```python
from build123d import *

# Parameters (mm, degrees)
SKETCH1_W           = 17
SKETCH1_H           = 10
BOSS_EXTRUDE1_DEPTH = 1
SKETCH2_W           = 3
SKETCH2_H           = 4
BOSS_EXTRUDE2_DEPTH = 1
SKETCH3_W           = 22.308498818
SKETCH3_H           = 11.48116176
SKETCH3_W_2         = 12.6
SKETCH3_H_2         = 7.6
CUT_EXTRUDE1_DEPTH  = 1
SKETCH4_R           = 0.5
SKETCH4_R_2         = 1.1
CUT_EXTRUDE2_DEPTH  = 1
SKETCH5_W           = 3.647171716
SKETCH5_H           = 4.834622973
SKETCH5_W_2         = 2.9
SKETCH5_H_2         = 3.6
CUT_EXTRUDE3_DEPTH  = 1


with BuildPart() as part:
    # Sketch1 → Boss-Extrude1 (new body)
    with BuildSketch(Plane(origin=(0, 0, 0), x_dir=(1, 0, 0), z_dir=(0, 1, 0))):
        with Locations((-16, 13.384146341)):
            Rectangle(SKETCH1_W, SKETCH1_H)
    extrude(amount=BOSS_EXTRUDE1_DEPTH)

    # Sketch2 → Boss-Extrude2 (add)
    with BuildSketch(Plane(origin=(0, 1, 0), x_dir=(1, 0, 0), z_dir=(0, 1, 0))):
        with Locations((-21, 13.384146341)):
            Rectangle(SKETCH2_W, SKETCH2_H)
    extrude(amount=BOSS_EXTRUDE2_DEPTH)

    # Sketch3 → Cut-Extrude1 (cut)
    with BuildSketch(Plane(origin=(0, 1, 0), x_dir=(1, 0, 0), z_dir=(0, 1, 0))):
        with Locations((-18.026856575, 13.593370246)):
            Rectangle(SKETCH3_W, SKETCH3_H)
        with Locations((-18.2, 13.384146341)):
            Rectangle(SKETCH3_W_2, SKETCH3_H_2, mode=Mode.SUBTRACT)
    extrude(amount=-CUT_EXTRUDE1_DEPTH, mode=Mode.SUBTRACT)

    # Sketch4 → Cut-Extrude2 (cut)
    with BuildSketch(Plane(origin=(0, 1, 0), x_dir=(1, 0, 0), z_dir=(0, 1, 0))):
        with Locations((-23.5, 13.384146341)):
            Circle(SKETCH4_R)
        with Locations((-23.5, 15.924146341)):
            Circle(SKETCH4_R)
        with Locations((-23.5, 10.844146341)):
            Circle(SKETCH4_R)
        with Locations((-13.9, 13.384146341)):
            Circle(SKETCH4_R_2)
    extrude(amount=-CUT_EXTRUDE2_DEPTH, mode=Mode.SUBTRACT)

    # Sketch5 → Cut-Extrude3 (cut)
    with BuildSketch(Plane(origin=(0, 2, 0), x_dir=(1, 0, 0), z_dir=(0, 1, 0))):
        with Locations((-20.925831492, 13.474507318)):
            Rectangle(SKETCH5_W, SKETCH5_H)
        with Locations((-21, 13.384146341)):
            Rectangle(SKETCH5_W_2, SKETCH5_H_2, mode=Mode.SUBTRACT)
    extrude(amount=-CUT_EXTRUDE3_DEPTH, mode=Mode.SUBTRACT)


solid = part.part
```
CAD build for the part. Positions are in the model's coordinates, mm. A direction names the side the tool comes from. Coordinates: 2 decimals unless noted, no trailing zeros. Order: outer loops, then holes, each group sorted by start corner. A loop starts at its lowest first (then second) coordinate and runs counter-clockwise, first axis right, second up. Notation, with made-up numbers: M 3,35.5 L 35,35.5 A30 ccw 35,65.5 Z; hole C -8,-26 d7. An arc over 180 degrees is marked long. Answer as CSV lines item,"result".
1) Mould opens along X. For faces 1 (the flat face through (-18.3, 0.5, -9.584)), 2 (the cylindrical face through (-13.39, 0.51, -12.41)), 3 (the flat face through (-22.45, 1.5, -13.4)), 4 (the flat face through (-19.55, 1.5, -13.4)) say: released by +X, released by -X, zero draft, split by the parting line, or undercut.
Verdict:
face 1,"zero draft"
face 2,"undercut"
face 3,"released by -X"
face 4,"released by +X"
2) Cut at B-B (x = -23.5). List the corners of the cut face in (y, z), then the cut area to 3 significant figures.
Verdict:
outline,"M 0,-17.18 L 1,-17.18 L 1,-16.42 L 0,-16.42 Z; M 0,-15.42 L 1,-15.42 L 1,-13.88 L 0,-13.88 Z; M 0,-12.88 L 1,-12.88 L 1,-11.34 L 0,-11.34 Z; M 0,-10.34 L 1,-10.34 L 1,-9.58 L 0,-9.58 Z"
area,"4.60 mm2"
3) Drill centre lines: L1, parallel to Z at x = -23.5, y = 0.65; L2, parallel to X at y = 0.6, z = -13.25; L3, parallel to Z at x = -13.9, y = 0.4. Where is each one in solid material? Low to high. Write a range as from..to.
Verdict:
L1,"-17.18..-16.42, -15.42..-13.88, -12.88..-11.34, -10.34..-9.58"
L2,"-24.5..-23.98, -23.02..-14.99, -12.81..-11.9"
L3,"-17.18..-14.48, -12.28..-9.58"
4) Cut at C-C (z = -10.5). List the corners of the cut face in (x, y).
Verdict:
outline,"M -24.5,0 L -23.86,0 L -23.86,1 L -24.5,1 Z; M -23.14,0 L -11.9,0 L -11.9,1 L -23.14,1 Z"
5) Flat gauge pins, fed straight in: P1, Ø4, axis at x = -14, z = -13.5, coming from the +Y side; P2, Ø0.8, axis at y = 1.5, z = -13.5, coming from the -X side; P3, Ø0.8, axis at y = 1.5, z = -13, coming from the +X side. Where does each tip first touch, or does it go through?
Verdict:
P1,"y = 1"
P2,"x = -22.45"
P3,"x = -19.55"
6) Cut at A-A (x = -13.9). List the corners of the cut face in (y, z).
Verdict:
outline,"M 0,-17.18 L 1,-17.18 L 1,-14.48 L 0,-14.48 Z; M 0,-12.28 L 1,-12.28 L 1,-9.58 L 0,-9.58 Z"
7) Cut at D-D (y = 0.6). List the corners of the cut face in (x, z).
Verdict:
outline,"M -24.5,-17.18 L -11.9,-17.18 L -11.9,-9.58 L -24.5,-9.58 Z; hole C -23.5,-15.92 d1; hole C -23.5,-13.38 d1; hole C -23.5,-10.84 d1; hole C -13.9,-13.38 d2.2"
8) 3-axis set-ups, long thin cutter, end or side, ignore diameter. For faces 5 (the flat face through (-18.3, 0.5, -17.184)), 6 (the flat face through (-21, 1.5, -15.184)), 7 (the flat face through (-21, 1.5, -11.584)): which of +Z, -Z, +X, -X, +Y, -Y reach the whole face in a straight line?
Verdict:
face 5,"-Z, +X, -X, +Y, -Y"
face 6,"-Z, +X, -X, +Y"
face 7,"+Z, +X, -X, +Y"
